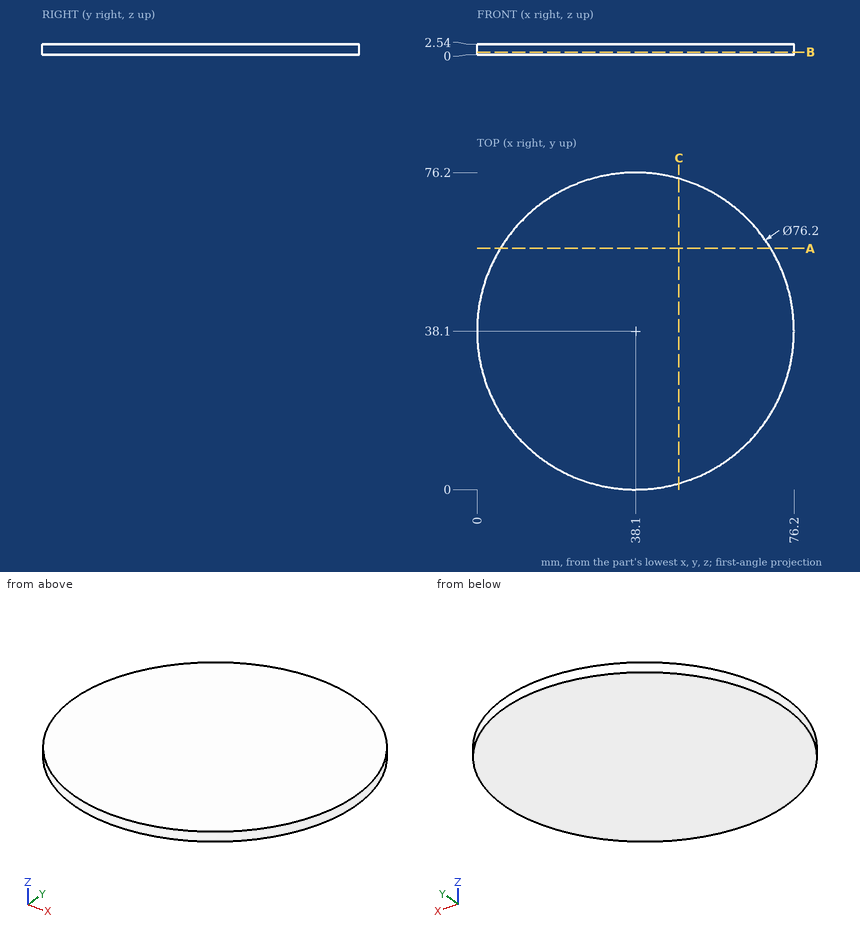
Print and shaded views of the part. All mm, measured from the part's lowest x, y and z. Coordinates: 2 decimals unless noted, no trailing zeros. Order: outer loops, then holes, each group sorted by start corner. A loop starts at its lowest first (then second) coordinate and runs counter-clockwise, first axis right, second up. Notation, with made-up numbers: M 55.25,46 L 112.25,46 A18 cw 112.25,77 Z; hole C 23.25,75.5 d1. An arc over 180 degrees is marked long. One line per question, with ' | ' between items. Start each with the question number.
Q1. Saw through at C-C (x = 48.5). List the corners of the cut face in (y, z), then the cut area to 3 significant figures.
Q2. Saw through at B-B (z = 0.6). List the corners of the cut face in (x, y).
Q3. Flat gauge pins, fed straight in: pin 1 Ø1.5 at (y, z) = (64, 1) entering from -X; pin 2 Ø1.5 at (y, z) = (55, 2) entering from -X. Where does each tip first touch, or does it go through?
Q4. Probe L1, parallel to Y at x = 37.5, z = 0.2; L2, parallel to X at y = 27, z = 0.7; L3, parallel to X at y = 35.5, z = 1.2. List the from-to ranges inside material, lowest first. Write a range as from..to.
Q5. Saw through at A-A (y = 58). List the corners of the cut face in (x, z), then the cut area to 3 significant figures.
Check values:
1) outline: M 1.45,0 L 74.75,0 L 74.75,2.54 L 1.45,2.54 Z | area: 186 mm2
2) outline: C 38.1,38.1 d76.2
3) pin 1: stops at x = 9.48 | pin 2: stops at x = 3.59
4) L1: y = 0..76.2 | L2: x = 1.65..74.55 | L3: x = 0.09..76.11
5) outline: M 5.61,0 L 70.59,0 L 70.59,2.54 L 5.61,2.54 Z | area: 165 mm2
